Here's how the part is built. I have some questions about the finished solid (model axes, mm). A direction names the side the tool comes from. Round coordinates to 2 decimals unless told otherwise and drop trailing zeros. Loops run counter-clockwise (first coordinate to the right, second up) from the corner with the lowest first, then second, coordinate; pieces in that order, holes last. Notation, with made-up numbers: M -13,36 L 38,36 A32 ccw 38,67 Z; hole C 1.5,61 d9. An arc over 180 degrees is marked long. Answer as CSV lines item,"result".
```python
from build123d import *

# Parameters (mm, degrees)
CHANFREIN1_SIZE = 0.3


with BuildPart() as part:
    # Esquisse1 → Révolution1 (revolve)
    with BuildSketch(Plane.XY, mode=Mode.PRIVATE) as r_volution1_sk:
        Polygon((-2.5, 0), (-2.5, 4.5), (-5, 4.5), (-5, 1.25), (-4, 1.25), (-4, 0), align=None)
    revolve(r_volution1_sk.sketch.rotate(Axis((0, 0, 0), (0, 1, 0)), 270), axis=Axis((0, 0, 0), (0, 1, 0)))  # turned: the seam where the file's is

    # Chanfrein1
    chanfrein1_edges = [part.edges().sort_by_distance(p)[0] for p in [
        (0, 1.25, 5),
        (0, 4.5, 5),
    ]]
    chamfer(chanfrein1_edges, length=CHANFREIN1_SIZE)


solid = part.part
```
1. Which directions (+Z, -Z, +X, -X, +Y, -Y) give clear straight access to the entire face, cutting with the end or side of a thin tool? Please do faces 4 (the flat face through (-4, 1.25, -2)), 5 (the flat face through (2, 4.5, 2)).
Evaluation:
face 4,"-Y"
face 5,"+Z, -Z, +X, -X, +Y"
2. I want a section at A-A, the plane x = 0. Please give me the cut outline in (y, z), and give its area (3 significant figures).
Evaluation:
outline,"M 0,-4 L 1.25,-4 L 1.25,-4.7 L 1.55,-5 L 4.2,-5 L 4.5,-4.7 L 4.5,-2.5 L 0,-2.5 Z; M 0,2.5 L 4.5,2.5 L 4.5,4.7 L 4.2,5 L 1.55,5 L 1.25,4.7 L 1.25,4 L 0,4 Z"
area,"19.8 mm²"
3. I want a section at D-D, the plane y = 3.3. Please give me the cut outline in (x, z), and give its area (3 significant figures).
Evaluation:
outline,"C 0,0 d10; hole C 0,0 d5"
area,"58.9 mm²"
4. We'd pull the mould along Z, two halves only. Please class faces 1 (the flat face through (-2, 0, -2)), 2 (the cylindrical face through (4.88, 2.86, 1.08)), 3 (the cylindrical face through (2.44, 2.28, 0.54)): pulls with the +Z half, pulls with the -Z half, needs draft (parallel to the pull), parting line crosses it, or undercut.
Evaluation:
face 1,"needs draft"
face 2,"parting line crosses it"
face 3,"undercut"
5. I want a section at B-B, the plane z = 0. Please give me the cut outline in (x, y), and give its area (3 significant figures).
Evaluation:
outline,"M -5,1.55 L -4.7,1.25 L -4,1.25 L -4,0 L -2.5,0 L -2.5,4.5 L -4.7,4.5 L -5,4.2 Z; M 2.5,0 L 4,0 L 4,1.25 L 4.7,1.25 L 5,1.55 L 5,4.2 L 4.7,4.5 L 2.5,4.5 Z"
area,"19.8 mm²"
6. For P1, Ø2, axis at x = -4, y = 4, coming from the +Z side, with a flat end and sliding along its axis, tell me the tip position at first contact or that it passes through.
Evaluation:
P1,"stops at z = 4"
7. I want a section at C-C, the plane y = 0.55. Please give me the cut outline in (x, z).
Evaluation:
outline,"C 0,0 d8; hole C 0,0 d5"
8. If I drill on line 1 (X direction, y = 3, z = 0); line 2 (Y direction, x = -4, z = -1); line 3 (X direction, y = 1.35, z = 0.5), over which ranges is the centre line in solid material (lowest first)? Write a range as [from, to].
Evaluation:
line 1,"x = [-5, -2.5], [2.5, 5]"
line 2,"y = [1.25, 4.5]"
line 3,"x = [-4.77, -2.45], [2.45, 4.77]"
